Source: CAD feature listing. Evaluate the final solid. Frame: model axes, mm. Face numbers are marked on the shaded views. A direction names the side the tool comes from. Round coordinates to 2 decimals unless told otherwise and drop trailing zeros. Write each loop counter-clockwise with the first axis right and the second up, starting at its lowest first coordinate (ties: lowest second). Pieces come first, ordered by that corner, then holes. Notation, with made-up numbers: (46, 45.25) -> (103, 45.25) arc R25 cw to (103, 83.25) -> close; hole circle Ø7 at (63.25, -21.5). An arc over 180 degrees is marked (long way). Return JSON: item names as keys, results as strings. Group by question number.
from build123d import *

# Parameters (mm, degrees)
SKETCH_1_W               = 18
SKETCH_1_H               = 27.5
SKETCH_1_R               = 2.5
TOP_SURFACE_DEPTH        = 3.5
SKETCH_2_R               = 1.7
FRONT_WALL_DEPTH         = 2
PATTERN_CIRCULAR_1_COUNT = 2
SIDE_RAILS_DEPTH         = 27.5
SKETCH_4_R               = 1
SEPARATORS_CUTOUTS_DEPTH = 9
PATTERN_CIRCULAR_5_COUNT = 2


with BuildPart() as part:
    # Эскиз1 → top-surface (new body)
    with BuildSketch(Plane(origin=(0, 0, 0), x_dir=(1, 0, 0), z_dir=(0, 1, 0))):
        Rectangle(SKETCH_1_W, SKETCH_1_H)
        with Locations(Location((-4, 7.25, 0), (0, 0, 270))):
            Circle(SKETCH_1_R, mode=Mode.SUBTRACT)
        with Locations(Location((-4, -0.25, 0), (0, 0, 270))):
            Circle(SKETCH_1_R, mode=Mode.SUBTRACT)
        with Locations(Location((-4, -7.75, 0), (0, 0, 270))):
            Circle(SKETCH_1_R, mode=Mode.SUBTRACT)
        with BuildLine():
            Line((2.5, 9.25), (5.5, 9.25))
            ThreePointArc((5.5, 9.25), (4, 4.75), (2.5, 9.25))
        make_face(mode=Mode.SUBTRACT)
        with BuildLine():
            Line((2.5, 1.75), (5.5, 1.75))
            ThreePointArc((5.5, 1.75), (4, -2.75), (2.5, 1.75))
        make_face(mode=Mode.SUBTRACT)
        with BuildLine():
            Line((2.5, -5.75), (5.5, -5.75))
            ThreePointArc((5.5, -5.75), (4, -10.25), (2.5, -5.75))
        make_face(mode=Mode.SUBTRACT)
    extrude(amount=-TOP_SURFACE_DEPTH)

    # Эскиз2 → front-wall (add)
    with BuildSketch(Plane.XY.offset(13.75)):
        with BuildLine():
            Line((9, -3.5), (-9, -3.5))
            Line((-9, -3.5), (-9, -22))
            Line((-9, -22), (-5.7, -22))
            Line((-5.7, -22), (-5.7, -16))
            ThreePointArc((-5.7, -16), (-4, -14.3), (-2.3, -16))
            Line((-2.3, -16), (-2.3, -22))
            Line((-2.3, -22), (9, -22))
            Line((9, -22), (9, -3.5))
        make_face()
        with Locations((4, -16)):
            Circle(SKETCH_2_R, mode=Mode.SUBTRACT)
    front_wall = extrude(amount=-FRONT_WALL_DEPTH)

    # Круговой массив1: front-wall ×2 about axis
    pattern_circular_1_axis = Axis((0, 0, 0), (0, 1, 0))
    for i in range(1, PATTERN_CIRCULAR_1_COUNT):
        add(front_wall.rotate(pattern_circular_1_axis, i * 360 / PATTERN_CIRCULAR_1_COUNT))

    # Эскиз5 → side-rails (add)
    with BuildSketch(Plane.XY.offset(13.75)):
        Polygon((-9, -1.5), (-9, -11), (-7, -11), (-6.3, -10.3), (-6.3, -8.3), (-7, -7.6), (-7, -1.5), align=None)
        Polygon((-1.7, -8.3), (-1, -7.6), (-1, -1.5), (0, -1.5), (0, -11), (-1, -11), (-1.7, -10.3), align=None)
    side_rails = extrude(amount=-SIDE_RAILS_DEPTH)

    # Эскиз4 → separators-cutouts (cut)
    with BuildSketch(Plane.ZY.offset(9)):
        with Locations((-5, -9.3)):
            Circle(SKETCH_4_R)
        with Locations((2.5, -9.3)):
            Circle(SKETCH_4_R)
        with Locations((10, -9.3)):
            Circle(SKETCH_4_R)
    separators_cutouts = extrude(amount=-SEPARATORS_CUTOUTS_DEPTH, mode=Mode.SUBTRACT)

    # Круговой массив5: side-rails, separators-cutouts ×2 about axis
    pattern_circular_5_axis = Axis((0, 0, 0), (0, 1, 0))
    add([side_rails.rotate(pattern_circular_5_axis, i * 360 / PATTERN_CIRCULAR_5_COUNT) for i in range(1, PATTERN_CIRCULAR_5_COUNT)])
    add([separators_cutouts.rotate(pattern_circular_5_axis, i * 360 / PATTERN_CIRCULAR_5_COUNT) for i in range(1, PATTERN_CIRCULAR_5_COUNT)], mode=Mode.SUBTRACT)


solid = part.part
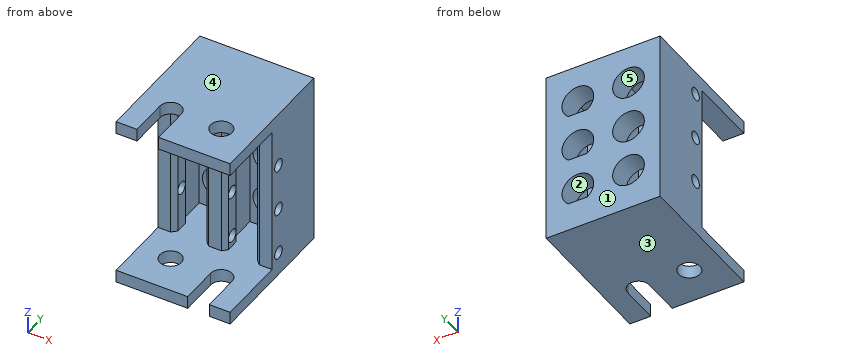
Item 1: Material intervals for probe 1 along Z at (x, y) = (4, -2.05); probe 2 along Z at (x, y) = (-7.05, -9.3); probe 3 along X at (y, z) = (-1.4, 7.75), sorted ascending.
Item 2: Cut plane C-C on y = -19.5. Output: boundary loops of the cut face in (x, z).
Item 3: Set-up query: the marked faces 4 and 5. Return all of +Z, -Z, +X, -X, +Y, -Y with unobstructed straight access to the full face (end or side cutting, diameter ignored); none if empty.
Item 4: Cut plane D-D on x = -4. Output: boundary loops of the cut face in (y, z), and give its area (4 significant figures).
Item 5: Cut plane B-B on y = -11.5. Output: boundary loops of the cut face in (x, z), and give its area (3 significant figures).
Item 6: Cut plane A-A on z = 7.75. Give the number of separate pieces and of enclosed holes in the cut face, and give its area (3 significant figures).
Item 7: First-contact query: pin 1 Ø1.2 at (y, z) = (-9.3, -2.5) entering from +X; pin 2 Ø6 at (x, z) = (5.5, 6) entering from -Y. Flat tips, straight axial feed; report the tip coordinate or a pass-through.
Item 8: Pull-direction query (Z, two-part tool) for the marked faces 1, 2 and 3; classes: +Z half, -Z half, draft (parallel to the pull), parting line (faces both ways), or undercut.
Here are the results:
{
 "1": {"probe 1": "z = -13.75 to -9.25, -4.75 to -1.75, 2.75 to 5.75, 10.25 to 13.75", "probe 2": "z = -13.75 to -6, -4 to 1.5, 3.5 to 9, 11 to 13.75", "probe 3": "x = -9 to -6.5, -1.5 to 1.5, 6.5 to 9"},
 "2": {"outline": "(-9, -13.75) -> (2.3, -13.75) -> (2.3, -11.75) -> (-9, -11.75) -> close; (-9, 11.75) -> (-5.7, 11.75) -> (-5.7, 13.75) -> (-9, 13.75) -> close; (-2.3, 11.75) -> (9, 11.75) -> (9, 13.75) -> (-2.3, 13.75) -> close; (5.7, -13.75) -> (9, -13.75) -> (9, -11.75) -> (5.7, -11.75) -> close"},
 "3": {"face 4": "+Z, +X, -X, +Y, -Y", "face 5": "+Y"},
 "4": {"outline": "(-22, -13.75) -> (-17.7, -13.75) -> (-17.7, -11.75) -> (-22, -11.75) -> close; (-14.3, -13.75) -> (0, -13.75) -> (0, -9.75) -> (-3.5, -9.75) -> (-3.5, -11.75) -> (-14.3, -11.75) -> close; (-14.3, 11.75) -> (-3.5, 11.75) -> (-3.5, 10.25) -> (0, 10.25) -> (0, 13.75) -> (-14.3, 13.75) -> close; (-3.5, -4.75) -> (0, -4.75) -> (0, -2.25) -> (-3.5, -2.25) -> close; (-3.5, 2.75) -> (0, 2.75) -> (0, 5.25) -> (-3.5, 5.25) -> close", "area": "95.55 mm^2"},
 "5": {"outline": "(-9, -13.75) -> (9, -13.75) -> (9, -11.75) -> (-9, -11.75) -> close; (-9, 11.75) -> (9, 11.75) -> (9, 13.75) -> (-9, 13.75) -> close", "area": "72.0 mm^2"},
 "6": {"separate pieces": "3", "enclosed holes": "0", "area": "80.6 mm^2"},
 "7": {"pin 1": "stops at x = 0", "pin 2": "stops at y = -11"},
 "8": {"face 1": "draft", "face 2": "undercut", "face 3": "-Z half"}
}
